Verification items for this drawing (mm, ordinates from the low corner). Round coordinates to 2 decimals unless told otherwise and drop trailing zeros. Loops run counter-clockwise (first coordinate to the right, second up) from the corner with the lowest first, then second, coordinate; pieces in that order, holes last. Notation, with made-up numbers: (-33, 40.5) - (-8, 40.5) arc R20 ccw to (-8, 77.5) - close; hole circle Ø7 at (-12, 50). An arc over 180 degrees is marked (long way). Answer in a Markdown table with one row per item. Add a question column.
(1) Cross-section at B-B on z = 12.7. Enter the section's corners in (x, y) (3 decimals), then the cut area to 3 significant figures.
(2) Cross-section at A-A on z = 38.1. Enter the section's corners in (x, y) (3 decimals), then the cut area to 3 significant figures.
(3) Cross-section at D-D on z = 62.5. Enter the section's corners in (x, y) (3 decimals), then the cut area to 3 significant figures.
(4) Thickness scan on line 1 along X through (y, z) = (0.6, 63); line 2 along X through (y, z) = (1.4, 88.9) (3 decimals); line 3 along Z through (x, y) = (114.3, 1.1) (3 decimals). Record the ranges inside material, lowest first.
(5) Cross-section at C-C on y = 0.7. Count the separate pieces of the cut face and the enclosed holes in it, then the cut area to 3 significant figures.
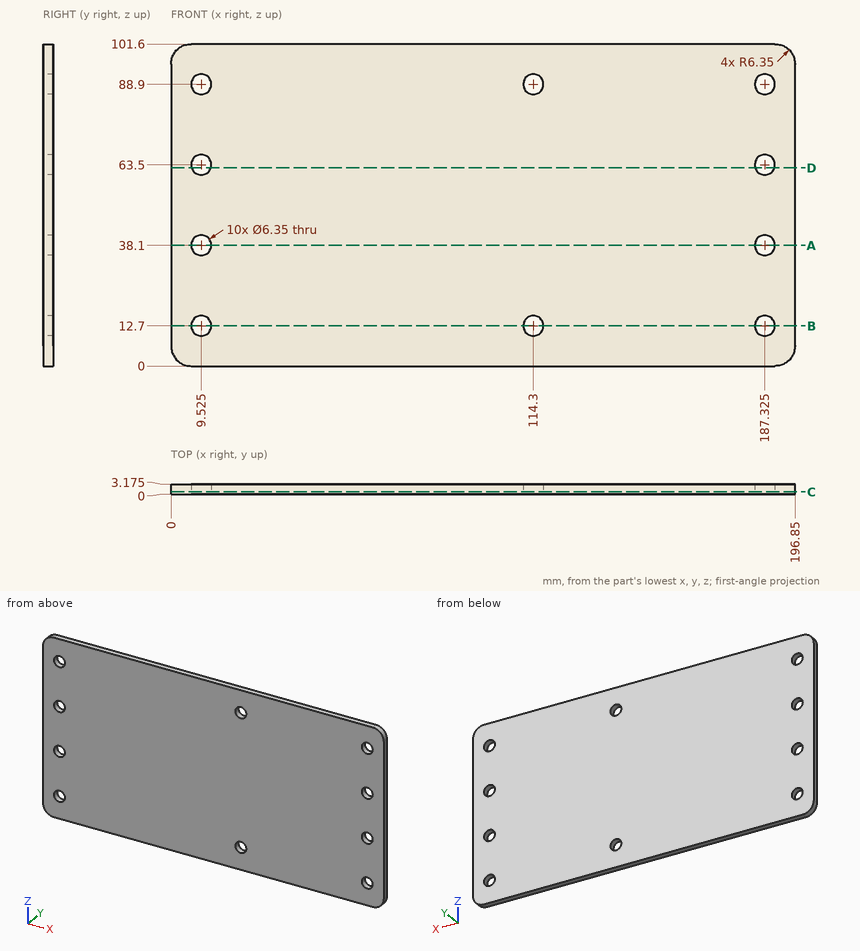
Answers:
| question | item | result |
|---|---|---|
| 1 | outline | (0, 0) - (6.35, 0) - (6.35, 3.175) - (0, 3.175) - close; (12.7, 0) - (111.125, 0) - (111.125, 3.175) - (12.7, 3.175) - close; (117.475, 0) - (184.15, 0) - (184.15, 3.175) - (117.475, 3.175) - close; (190.5, 0) - (196.85, 0) - (196.85, 3.175) - (190.5, 3.175) - close |
| 1 | area | 565 mm^2 |
| 2 | outline | (0, 0) - (6.35, 0) - (6.35, 3.175) - (0, 3.175) - close; (12.7, 0) - (184.15, 0) - (184.15, 3.175) - (12.7, 3.175) - close; (190.5, 0) - (196.85, 0) - (196.85, 3.175) - (190.5, 3.175) - close |
| 2 | area | 585 mm^2 |
| 3 | outline | (0, 0) - (6.512, 0) - (6.512, 3.175) - (0, 3.175) - close; (12.538, 0) - (184.312, 0) - (184.312, 3.175) - (12.538, 3.175) - close; (190.338, 0) - (196.85, 0) - (196.85, 3.175) - (190.338, 3.175) - close |
| 3 | area | 587 mm^2 |
| 4 | line 1 | x = 0 to 6.39, 12.66 to 184.19, 190.46 to 196.85 |
| 4 | line 2 | x = 0 to 6.35, 12.7 to 111.125, 117.475 to 184.15, 190.5 to 196.85 |
| 4 | line 3 | z = 0 to 9.525, 15.875 to 85.725, 92.075 to 101.6 |
| 5 | separate pieces | 1 |
| 5 | enclosed holes | 10 |
| 5 | area | 19,600 mm^2 |
